Input: part model. Units: mm. Frame: model coordinates. A direction names the side the tool comes from. Coordinates: 2 decimals unless noted, no trailing zeros. Write each loop counter-clockwise with the first axis right and the second up, starting at its lowest first coordinate (ties: lowest second). Pieces come first, ordered by that corner, then holes. Notation, with made-up numbers: (-25.5, -38.75) -> (33.5, -38.75) arc R24 cw to (33.5, -20.75) -> close; hole circle Ø4 at (67, 59.5). An arc over 180 degrees is marked (long way). Use one line per item in the form item = value. Start each with the question number.
(1) Cut plane B-B on x = 18. Return the cut outline in (y, z), plus the area to 3 significant figures.
(2) Pull-direction query (Z, two-part tool) for faces 1 (the face through (31.868, 55.768, 13.244)), 2 (the face through (29, 53, 5)), 3 (the face through (7, 50, 0)), 4 (the face through (-20, 31, -28)); classes: released by +Z, released by -Z, zero draft, split by the parting line, or undercut.
(3) Set-up query: faces 5 (the face through (25.9, 55.77, 31.76)), 6 (the face through (23, 53, 20)), 7 (the face through (-23, 31, -25)). Return all of +Z, -Z, +X, -X, +Y, -Y with unobstructed straight access to the full face (end or side cutting, diameter ignored); none if empty.
(4) Cut plane C-C on z = 41.5. Return the cut outline in (x, y), plus the area to 3 significant figures.
(5) Cut plane D-D on y = 24.5. Return the cut outline in (x, z), plus the area to 3 significant figures.
(6) First-contact query: pin 1 (3.5 mm diameter, centred on y = 54, z = 20, fed in from -X); pin 2 (3 mm diameter, centred on x = 28.5, z = 15.5, fed in from +Y); pin 3 (1 mm diameter, centred on x = 4.5, y = 34, fed in from +Z); pin 4 (10 mm diameter, centred on x = -12, z = -8.5, fed in from -Y). Flat tips, straight axial feed; report the tip coordinate or a pass-through.
(7) Ray query, line 1 along X through (y, z) = (40.75, 15); line 2 along Z through (x, y) = (30, 2); line 3 along Z through (x, y) = (10.5, 21). Return the intervals inside material, ascending.
(8) Cut plane A-A on z = 20. Return the cut outline in (x, y).
```python
from build123d import *

# Parameters (mm, degrees)
SKETCH1_W           = 70
SKETCH1_H           = 70
BOSS_EXTRUDE1_DEPTH = 50
CUT_EXTRUDE1_DEPTH  = 40
SKETCH3_W           = 20
SKETCH3_H           = 41
CUT_EXTRUDE2_DEPTH  = 40
SKETCH4_W           = 12
SKETCH4_H           = 30
BOSS_EXTRUDE2_DEPTH = 7
CUT_EXTRUDE3_DEPTH  = 2.5
SKETCH7_R           = 2.5
CUT_EXTRUDE4_DEPTH  = 52.5
SKETCH10_W          = 10
SKETCH10_H          = 6
CUT_EXTRUDE6_DEPTH  = 55
SKETCH11_W          = 20
SKETCH11_H          = 10
BOSS_EXTRUDE3_DEPTH = 12
SKETCH13_W          = 10
SKETCH13_H          = 5
BOSS_EXTRUDE4_DEPTH = 13
SKETCH14_W          = 10
SKETCH14_H          = 5
BOSS_EXTRUDE5_DEPTH = 13
SKETCH15_R          = 3
CUT_EXTRUDE7_DEPTH  = 33
CUT_EXTRUDE8_DEPTH  = 10
SKETCH18_R          = 1.75
CUT_EXTRUDE9_DEPTH  = 20


with BuildPart() as part:
    # Sketch1 → Boss-Extrude1 (new body)
    with BuildSketch(Plane(origin=(0, 0, 0), x_dir=(1, 0, 0), z_dir=(0, 1, 0))):
        Rectangle(SKETCH1_W, SKETCH1_H)
    extrude(amount=BOSS_EXTRUDE1_DEPTH)

    # Sketch2 → Cut-Extrude1 (cut)
    with BuildSketch(Plane.XZ):
        Polygon((0, 25), (-25, 25), (-25, -25), (25, -25), (25, 25), align=None)
    extrude(amount=-CUT_EXTRUDE1_DEPTH, mode=Mode.SUBTRACT)

    # Sketch3 → Cut-Extrude2 (cut)
    with BuildSketch(Plane(origin=(0, 50, 0), x_dir=(1, 0, 0), z_dir=(0, 1, 0))):
        with Locations((-15, 4.5)):
            Rectangle(SKETCH3_W, SKETCH3_H)
    extrude(amount=-CUT_EXTRUDE2_DEPTH, mode=Mode.SUBTRACT)

    # Sketch4 → Boss-Extrude2 (add)
    with BuildSketch(Plane(origin=(0, 50, 0), x_dir=(1, 0, 0), z_dir=(0, 1, 0))):
        with Locations((29, -20)):
            Rectangle(SKETCH4_W, SKETCH4_H)
    extrude(amount=BOSS_EXTRUDE2_DEPTH)

    # Sketch5 → Cut-Extrude3 (cut)
    with BuildSketch(Plane(origin=(0, 57, 0), x_dir=(1, 0, 0), z_dir=(0, 1, 0))):
        Polygon((32.881686691, -15), (30.881686691, -18.464101615), (26.881686691, -18.464101615), (24.881686691, -15), (26.881686691, -11.535898385), (30.881686691, -11.535898385), align=None)
        Polygon((26.881686691, -33.464101615), (24.881686691, -30), (26.881686691, -26.535898385), (30.881686691, -26.535898385), (32.881686691, -30), (30.881686691, -33.464101615), align=None)
    extrude(amount=-CUT_EXTRUDE3_DEPTH, mode=Mode.SUBTRACT)

    # Sketch7 → Cut-Extrude4 (cut)
    with BuildSketch(Plane(origin=(0, 50, 0), x_dir=(1, 0, 0), z_dir=(0, 1, 0))):
        with Locations(Location((18, -20, 0), (0, 0, 270))):
            Circle(SKETCH7_R)
    extrude(amount=-CUT_EXTRUDE4_DEPTH, mode=Mode.SUBTRACT)

    # Sketch10 → Cut-Extrude6 (cut)
    with BuildSketch(Plane.XZ):
        with Locations((-15, -28)):
            Rectangle(SKETCH10_W, SKETCH10_H)
    extrude(amount=-CUT_EXTRUDE6_DEPTH, mode=Mode.SUBTRACT)

    # Sketch11 → Boss-Extrude3 (add)
    with BuildSketch(Plane(origin=(0, 50, 0), x_dir=(1, 0, 0), z_dir=(0, 1, 0))):
        Polygon((-25, 35), (-25, 25), (-20, 25), (-20, 31), (-10, 31), (-10, 25), (-5, 25), (-5, 35), align=None)
        with Locations((-15, -21)):
            Rectangle(SKETCH11_W, SKETCH11_H)
    extrude(amount=BOSS_EXTRUDE3_DEPTH)

    # Sketch13 → Boss-Extrude4 (add)
    with BuildSketch(Plane.XY.offset(35)):
        with Locations((-30, 2.5)):
            Rectangle(SKETCH13_W, SKETCH13_H)
        with Locations((30, 2.5)):
            Rectangle(SKETCH13_W, SKETCH13_H)
    extrude(amount=BOSS_EXTRUDE4_DEPTH)

    # Sketch14 → Boss-Extrude5 (add)
    with BuildSketch(Plane(origin=(0, 0, -35), x_dir=(-1, 0, 0), z_dir=(0, 0, -1))):
        with Locations((-30, 2.5)):
            Rectangle(SKETCH14_W, SKETCH14_H)
        with Locations((30, 2.5)):
            Rectangle(SKETCH14_W, SKETCH14_H)
    extrude(amount=BOSS_EXTRUDE5_DEPTH)

    # Sketch15 → Cut-Extrude7 (cut)
    with BuildSketch(Plane(origin=(0, 5, 0), x_dir=(1, 0, 0), z_dir=(0, 1, 0))):
        with Locations(Location((-29.888443239, 41.354976211, 0), (0, 0, 180))):
            Circle(SKETCH15_R)
        with Locations(Location((-30, -41.5, 0), (0, 0, 180))):
            Circle(SKETCH15_R)
        with Locations(Location((30, -41.5, 0), (0, 0, 180))):
            Circle(SKETCH15_R)
        with Locations(Location((30, 41.5, 0), (0, 0, 180))):
            Circle(SKETCH15_R)
    extrude(amount=-CUT_EXTRUDE7_DEPTH, mode=Mode.SUBTRACT)

    # Sketch16 → Cut-Extrude8 (cut)
    with BuildSketch(Plane.ZY.offset(35)):
        Polygon((-10, 0), (-10, 10), (-15, 10), (-20, 10), (-20, 0), align=None)
    extrude(amount=-CUT_EXTRUDE8_DEPTH, mode=Mode.SUBTRACT)

    # Sketch18 → Cut-Extrude9 (cut)
    with BuildSketch(Plane(origin=(0, 54.5, 0), x_dir=(1, 0, 0), z_dir=(0, 1, 0))):
        with Locations(Location((28.881686691, -15, 0), (0, 0, 270))):
            Circle(SKETCH18_R)
        with Locations(Location((28.881686691, -30, 0), (0, 0, 270))):
            Circle(SKETCH18_R)
    extrude(amount=-CUT_EXTRUDE9_DEPTH, mode=Mode.SUBTRACT)


solid = part.part
```
Values:
q1.outline = (0, -35) -> (50, -35) -> (50, 17.5) -> (40, 17.5) -> (40, -25) -> (0, -25) -> close; (0, 25) -> (40, 25) -> (40, 22.5) -> (50, 22.5) -> (50, 35) -> (0, 35) -> close
q1.area = 1,450 mm2
q2.face_1 = undercut
q2.face_2 = released by -Z
q2.face_3 = zero draft
q2.face_4 = undercut
q3.face_5 = +Y
q3.face_6 = +Z, -Z, +Y
q3.face_7 = +Y, -Y
q4.outline = (-35, 0) -> (-33, 0) -> (-33, 5) -> (-35, 5) -> close; (-27, 0) -> (-25, 0) -> (-25, 5) -> (-27, 5) -> close; (25, 0) -> (27, 0) -> (27, 5) -> (25, 5) -> close; (33, 0) -> (35, 0) -> (35, 5) -> (33, 5) -> close
q4.area = 40.0 mm2
q5.outline = (-35, -35) -> (35, -35) -> (35, 35) -> (-35, 35) -> close; hole (-25, -25) -> (-20, -25) -> (-20, -31) -> (-10, -31) -> (-10, -25) -> (25, -25) -> (25, 25) -> (-25, 25) -> close
q5.area = 2,340 mm2
q6.pin_1 = -25
q6.pin_2 = 54.5
q6.pin_3 = 35
q6.pin_4 = through
q7.line_1 = -35 to -25, -5 to 27.13, 30.63 to 35
q7.line_2 = -48 to -44.5, -38.5 to 38.5, 44.5 to 48
q7.line_3 = -35 to -25, 25 to 35
q8.outline = (-35, 0) -> (-25, 0) -> (-25, 40) -> (15.5, 40) -> (15.5, 50) -> (-5, 50) -> (-5, 62) -> (-25, 62) -> (-25, 50) -> (-35, 50) -> close; (20.5, 40) -> (25, 40) -> (25, 0) -> (35, 0) -> (35, 57) -> (23, 57) -> (23, 50) -> (20.5, 50) -> close
